```python
from build123d import *

# Parameters (mm, degrees)
SKETCH1_W           = 76.2
SKETCH1_H           = 500
BOSS_EXTRUDE2_DEPTH = 12.7
SKETCH3_W           = 70
SKETCH3_H           = 30
CUT_EXTRUDE4_DEPTH  = 6.604
LPATTERN1_COUNT     = 10
LPATTERN1_PITCH     = 50
SKETCH4_W           = 12.7
SKETCH4_H           = 500
BOSS_EXTRUDE4_DEPTH = 40
SKETCH5_W           = 30
SKETCH5_H           = 70
CUT_EXTRUDE5_DEPTH  = 6.604


with BuildPart() as part:
    # Sketch1 → Boss-Extrude2 (new body)
    with BuildSketch(Plane.XY):
        Rectangle(SKETCH1_W, SKETCH1_H)
    extrude(amount=BOSS_EXTRUDE2_DEPTH)

    # Sketch3 → Cut-Extrude4 (cut)
    with BuildSketch(Plane.XY.offset(12.7)):
        with Locations((0.129688718, 221.422286077)):
            Rectangle(SKETCH3_W, SKETCH3_H)
    cut_extrude4 = extrude(amount=-CUT_EXTRUDE4_DEPTH, mode=Mode.SUBTRACT)

    # LPattern1: Cut-Extrude4 ×10
    with Locations(*[(0, -i * LPATTERN1_PITCH, 0) for i in range(1, LPATTERN1_COUNT)]):
        add(cut_extrude4, mode=Mode.SUBTRACT)

    # Sketch4 → Boss-Extrude4 (add)
    with BuildSketch(Plane.ZY.offset(38.1)):
        with Locations((6.35, 0)):
            Rectangle(SKETCH4_W, SKETCH4_H)
    extrude(amount=BOSS_EXTRUDE4_DEPTH)

    # Sketch5 → Cut-Extrude5 (cut)
    with BuildSketch(Plane.XY.offset(12.7)):
        with Locations((-58.010071461, 23.936214581)):
            Rectangle(SKETCH5_W, SKETCH5_H)
    extrude(amount=-CUT_EXTRUDE5_DEPTH, mode=Mode.SUBTRACT)


solid = part.part
```
Build history of the part. All positions in model axes, mm. A direction names the side the tool comes from. Give positions to 0.01 mm unless a question says otherwise; leave off trailing zeros. Loops run counter-clockwise (first coordinate to the right, second up) from the corner with the lowest first, then second, coordinate; pieces in that order, holes last.
1) 3-axis set-ups, long thin cutter, end or side, ignore diameter. For faces 4 (the face through (-19, -250, 6)), 5 (the face through (0, 222, 6.096)): which of +Z, -Z, +X, -X, +Y, -Y reach the whole face in a straight line?
Values follow:
face 4: +Z, -Z, +X, -X, -Y
face 5: +Z
2) Probe line 1 along Y through (x, z) = (-52.5, 12.25); line 2 along X through (y, z) = (48, 11); line 3 along X through (y, z) = (160, 12). List the from-to ranges inside material, lowest first.
Values follow:
line 1: y = -250 to -11.06, 58.94 to 250
line 2: x = -78.1 to -73.01, -43.01 to 38.1
line 3: x = -78.1 to -34.87, 35.13 to 38.1
3) Band-saw the part on A-A on x = -64. List the corners of the cut face in (y, z), then the cut area to 3 significant figures.
Values follow:
outline: (-250, 0) - (250, 0) - (250, 12.7) - (58.94, 12.7) - (58.94, 6.1) - (-11.06, 6.1) - (-11.06, 12.7) - (-250, 12.7) - close
area: 5,890 mm2
4) Two-plate mould, pull along Y, no slides. Class faces 1 (the face through (-19, 250, 6)), 2 (the face through (0, 72, 6.096)), 3 (the face through (-19, -3, 0)): released by +Y, released by -Y, zero draft, split by the parting line, or undercut.
Values follow:
face 1: released by +Y
face 2: undercut
face 3: zero draft
5) Drop flat-ended pins along their axis: P1, Ø4, axis at x = -9.5, y = 126.5, coming from the +Z side; P2, Ø8, axis at x = -40, y = 78, coming from the -Z side. Give the stop position or say it passes through.
Values follow:
P1: stops at z = 6.1
P2: stops at z = 0
6) Band-saw the part on C-C on z = 10.5. State how many separate pieces and enclosed holes the cut face has, then the cut area to 3 significant figures.
Values follow:
separate pieces: 1
enclosed holes: 11
area: 35,000 mm2
7) Band-saw the part on B-B on y = 220. List the corners of the cut face in (x, z).
Values follow:
outline: (-78.1, 0) - (38.1, 0) - (38.1, 12.7) - (35.13, 12.7) - (35.13, 6.1) - (-34.87, 6.1) - (-34.87, 12.7) - (-78.1, 12.7) - close
